```python
from build123d import *

# Parameters (mm, degrees)
ESQUISSE1_R             = 1.5
BOSS_EXTRU_1_DEPTH      = 5
BOSS_EXTRU_2_START      = -1
ESQUISSE1_3_R           = 1.5
BOSS_EXTRU_2_DEPTH      = 1
ESQUISSE2_R             = 1.5
ENL_V_MAT_EXTRU_2_DEPTH = 28.129504234
ESQUISSE3_R             = 1.5
ENL_V_MAT_EXTRU_3_DEPTH = 21.182147001


with BuildPart() as part:
    # Esquisse1 → Boss.-Extru.1 (new body)
    with BuildSketch(Plane.XY):
        with BuildLine():
            Line((-9, 4.447944754), (-9, -4.447944754))
            ThreePointArc((-9, -4.447944754), (-8.756777021, -5.101617869), (-8.145422919, -5.437314339))
            ThreePointArc((-8.145422919, -5.437314339), (-6.252919377, -6.476494015), (-5.5, -8.5))
            Line((-5.5, -8.5), (-5.5, -11.715481211))
            ThreePointArc((-5.5, -11.715481211), (-5.324186186, -12.281800142), (-4.858565737, -12.64898569))
            ThreePointArc((-4.858565737, -12.64898569), (0, -13.55), (4.858565737, -12.64898569))
            ThreePointArc((4.858565737, -12.64898569), (5.324186186, -12.281800142), (5.5, -11.715481211))
            Line((5.5, -11.715481211), (5.5, 1.284668728))
            ThreePointArc((5.5, 1.284668728), (5.598803794, 1.718080078), (5.875690797, 2.065846057))
            ThreePointArc((5.875690797, 2.065846057), (7.096685887, 4.604672376), (5.875690797, 7.143498694))
            ThreePointArc((5.875690797, 7.143498694), (5.598803794, 7.491264673), (5.5, 7.924676023))
            Line((5.5, 7.924676023), (5.5, 11.715481211))
            ThreePointArc((5.5, 11.715481211), (5.324186186, 12.281800142), (4.858565737, 12.64898569))
            ThreePointArc((4.858565737, 12.64898569), (0, 13.55), (-4.858565737, 12.64898569))
            ThreePointArc((-4.858565737, 12.64898569), (-5.324186186, 12.281800142), (-5.5, 11.715481211))
            Line((-5.5, 11.715481211), (-5.5, 8.5))
            ThreePointArc((-5.5, 8.5), (-6.252919377, 6.476494015), (-8.145422919, 5.437314339))
            ThreePointArc((-8.145422919, 5.437314339), (-8.756777021, 5.101617869), (-9, 4.447944754))
        make_face()
        with Locations((-3.846685887, -4.604672376)):
            Circle(ESQUISSE1_R, mode=Mode.SUBTRACT)
        with Locations((3.846685887, 4.604672376)):
            Circle(ESQUISSE1_R, mode=Mode.SUBTRACT)
        with BuildLine():
            Line((-3.5, 11.55), (3.5, 11.55))
            Line((3.5, 11.55), (3.5, 8.5))
            ThreePointArc((3.5, 8.5), (0, 5), (-3.5, 8.5))
            Line((-3.5, 8.5), (-3.5, 11.55))
        make_face(mode=Mode.SUBTRACT)
        with BuildLine():
            Line((-3.5, -11.55), (3.5, -11.55))
            Line((3.5, -11.55), (3.5, -8.5))
            ThreePointArc((3.5, -8.5), (0, -5), (-3.5, -8.5))
            Line((-3.5, -8.5), (-3.5, -11.55))
        make_face(mode=Mode.SUBTRACT)
        with BuildLine():
            Line((0, -3), (-7, -3))
            Line((-7, -3), (-7, 3))
            Line((-7, 3), (0, 3))
            ThreePointArc((0, 3), (3, 0), (0, -3))
        make_face(mode=Mode.SUBTRACT)
    extrude(amount=BOSS_EXTRU_1_DEPTH)

    # Esquisse1_3 → Boss.-Extru.2 (add)
    with BuildSketch(Plane.XY.offset(BOSS_EXTRU_2_START)):
        with BuildLine():
            ThreePointArc((-8.145422919, 5.437314339), (-8.756777021, 5.101617869), (-9, 4.447944754))
            Line((-9, 4.447944754), (-9, -4.447944754))
            ThreePointArc((-9, -4.447944754), (-8.756777021, -5.101617869), (-8.145422919, -5.437314339))
            ThreePointArc((-8.145422919, -5.437314339), (-6.252919377, -6.476494015), (-5.5, -8.5))
            Line((-5.5, -8.5), (-5.5, -11.715481211))
            ThreePointArc((-5.5, -11.715481211), (-5.324186186, -12.281800142), (-4.858565737, -12.64898569))
            ThreePointArc((-4.858565737, -12.64898569), (0, -13.55), (4.858565737, -12.64898569))
            ThreePointArc((4.858565737, -12.64898569), (5.324186186, -12.281800142), (5.5, -11.715481211))
            Line((5.5, -11.715481211), (5.5, 1.284668728))
            ThreePointArc((5.5, 1.284668728), (5.598803794, 1.718080078), (5.875690797, 2.065846057))
            ThreePointArc((5.875690797, 2.065846057), (7.096685887, 4.604672376), (5.875690797, 7.143498694))
            ThreePointArc((5.875690797, 7.143498694), (5.598803794, 7.491264673), (5.5, 7.924676023))
            Line((5.5, 7.924676023), (5.5, 11.715481211))
            ThreePointArc((5.5, 11.715481211), (5.324186186, 12.281800142), (4.858565737, 12.64898569))
            ThreePointArc((4.858565737, 12.64898569), (0, 13.55), (-4.858565737, 12.64898569))
            ThreePointArc((-4.858565737, 12.64898569), (-5.324186186, 12.281800142), (-5.5, 11.715481211))
            Line((-5.5, 11.715481211), (-5.5, 8.5))
            ThreePointArc((-5.5, 8.5), (-6.252919377, 6.476494015), (-8.145422919, 5.437314339))
        make_face()
        with Locations((-3.846685887, -4.604672376)):
            Circle(ESQUISSE1_3_R, mode=Mode.SUBTRACT)
        with BuildLine():
            Line((3.5, 11.55), (3.5, 8.5))
            ThreePointArc((3.5, 8.5), (0, 5), (-3.5, 8.5))
            Line((-3.5, 8.5), (-3.5, 11.55))
            Line((-3.5, 11.55), (3.5, 11.55))
        make_face(mode=Mode.SUBTRACT)
        with Locations((3.846685887, 4.604672376)):
            Circle(ESQUISSE1_3_R, mode=Mode.SUBTRACT)
        with BuildLine():
            Line((3.5, -11.55), (-3.5, -11.55))
            Line((-3.5, -11.55), (-3.5, -8.5))
            ThreePointArc((-3.5, -8.5), (0, -5), (3.5, -8.5))
            Line((3.5, -8.5), (3.5, -11.55))
        make_face(mode=Mode.SUBTRACT)
    extrude(amount=BOSS_EXTRU_2_DEPTH)

    # Esquisse2 → Enl_v. mat.-Extru.2 (cut, through all)
    with BuildSketch(Plane.XZ.offset(-11.55)):
        with Locations(Location((0, 2, 0), (0, 0, 270))):
            Circle(ESQUISSE2_R)
    enl_v_mat_extru_2 = extrude(amount=-ENL_V_MAT_EXTRU_2_DEPTH, mode=Mode.SUBTRACT)

    # Sym_trie1: Enl_v. mat.-Extru.2 across plane
    add(enl_v_mat_extru_2.mirror(Plane.ZX), mode=Mode.SUBTRACT)

    # Esquisse3 → Enl_v. mat.-Extru.3 (cut, through all)
    with BuildSketch(Plane(origin=(-7, 0, 0), x_dir=(0, 0, -1), z_dir=(1, 0, 0))):
        with Locations((-2.5, 0)):
            Circle(ESQUISSE3_R)
    extrude(amount=-ENL_V_MAT_EXTRU_3_DEPTH, mode=Mode.SUBTRACT)


solid = part.part
```
Geometry check sheet. Reference: the model listing, model coordinates, mm. A direction names the side the tool comes from. Round coordinates to 2 decimals unless told otherwise and drop trailing zeros. Write each loop counter-clockwise with the first axis right and the second up, starting at its lowest first coordinate (ties: lowest second). Pieces come first, ordered by that corner, then holes. Notation, with made-up numbers: (14.25, 31.25) -> (19.25, 31.25) arc R15 ccw to (19.25, 52.25) -> close; hole circle Ø9 at (30, -16.5). An arc over 180 degrees is marked (long way). Put each result on its own line as item: value.
1) Cross-section at C-C, the plane y = -9. Enter the section's corners in (x, z), plus the area to 3 significant figures.
Recorded:
outline: (-5.5, -1) -> (-3.5, -1) -> (-3.5, 5) -> (-5.5, 5) -> close; (3.5, -1) -> (5.5, -1) -> (5.5, 5) -> (3.5, 5) -> close
area: 24.0 mm2
2) Access from +Z, -Z, +X, -X, +Y, -Y to the whole of each face (thin tool, end or side, straight path). Record for faces 1 (the face through (3.5, -10, 2)), 2 (the face through (-5.5, -10, 2)), 3 (the face through (5.5, 10, 2)).
Recorded:
face 1: +Z, -Z
face 2: +Z, -Z, -X, -Y
face 3: +Z, -Z, +X, +Y
3) Release check for a two-part mould opening along X. For faces 4 (the face through (-8.763, -5.094, 1.958)), 5 (the face through (0.45, 12.54, 0.57)), 6 (the face through (5.33, 12.27, 1.96)) record: pulls with the +X half, pulls with the -X half, needs draft (parallel to the pull), parting line crosses it, or undercut.
Recorded:
face 4: pulls with the -X half
face 5: undercut
face 6: pulls with the +X half
4) Thickness scan on probe 1 along X at (y, z) = (0, 4.75); probe 2 along Y at (x, z) = (-0.5, 3.75); probe 3 along X at (y, z) = (-11.25, 2.5). Record the ranges inside material, lowest first. Write a range as from..to.
Recorded:
probe 1: x = -9..-7, 3..5.5
probe 2: y = -13.54..-11.55, -5.04..-3, 3..5.04, 11.55..13.54
probe 3: x = -5.5..-3.5, 3.5..5.5
5) Depth check by flat-ended pin: P1, Ø2.5, axis at y = -10.5, z = 1, coming from the -X side; P2, Ø3.5, axis at y = -9.5, z = 3, coming from the +X side; P3, Ø1.8, axis at x = 0, z = 2, coming from the -Y side. Enter the tip coordinate at first touch or a pass-through.
Recorded:
P1: stops at x = -5.5
P2: stops at x = 5.5
P3: stops at y = -5.12
6) Cross-section at A-A, the plane y = 0. Enter the section's corners in (x, z).
Recorded:
outline: (-9, -1) -> (5.5, -1) -> (5.5, 5) -> (3, 5) -> (3, 0) -> (-7, 0) -> (-7, 1) -> (-9, 1) -> close; (-9, 4) -> (-7, 4) -> (-7, 5) -> (-9, 5) -> close
7) Cross-section at B-B, the plane x = -2. Enter the section's corners in (y, z).
Recorded:
outline: (-13.4, -1) -> (-11.55, -1) -> (-11.55, 5) -> (-13.4, 5) -> close; (-5.63, -1) -> (5.63, -1) -> (5.63, 5) -> (3, 5) -> (3, 0) -> (-3, 0) -> (-3, 5) -> (-5.63, 5) -> close; (11.55, -1) -> (13.4, -1) -> (13.4, 5) -> (11.55, 5) -> close
8) Cross-section at D-D, the plane x = -4.25. Enter the section's corners in (y, z).
Recorded:
outline: (-12.87, -1) -> (-6.05, -1) -> (-6.05, 5) -> (-12.87, 5) -> close; (-3.16, -1) -> (12.87, -1) -> (12.87, 5) -> (3, 5) -> (3, 0) -> (-3, 0) -> (-3, 5) -> (-3.16, 5) -> close
